Here's the drawing with two shaded views (mm, measured from the low corner). I have some questions. A direction names the side the tool comes from. Round coordinates to 2 decimals unless told otherwise and drop trailing zeros. Order: outer loops, then holes, each group sorted by start corner. A loop starts at its lowest first (then second) coordinate and runs counter-clockwise, first axis right, second up.
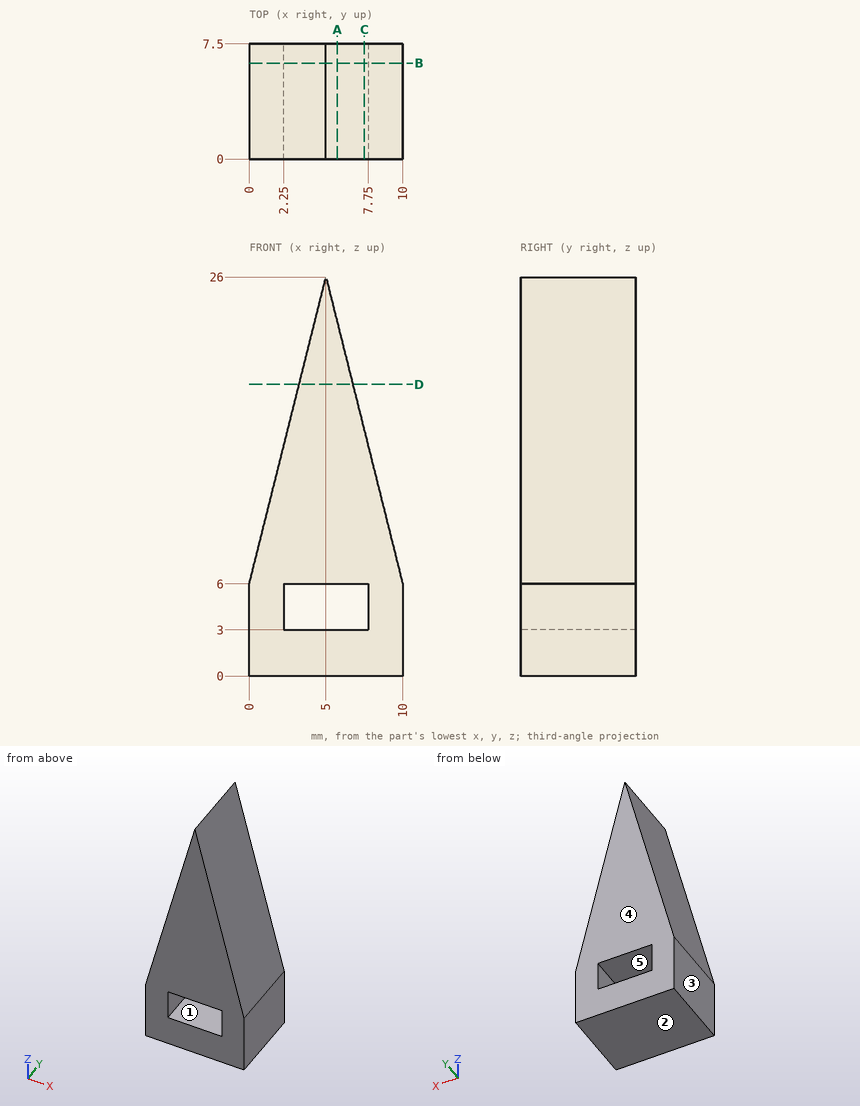
Q1. Imagine slicing it at A-A, the plane x = 5.75. Please give me the cut outline in (y, z), then the cut area to 3 significant figures.
Q2. I need wall thicknesses on L1, parallel to X at y = 5.75, z = 3.75; L2, parallel to X at y = 3.5, z = 15; L3, parallel to X at y = 1.25, z = 9.25. Which ranges of each line are inside material? Lowest first, please.
Q3. Imagine slicing it at D-D, the plane z = 19. Please give me the cut outline in (x, y).
Q4. We'd pull the mould along X, two halves only. Please class the marked faces 3, 4 and 5: released by +X, released by -X, zero draft, split by the parting line, or undercut.
Q5. For the marked faces 1 and 2, which set-ups out of +Z, -Z, +X, -X, +Y, -Y let a thin tool reach every point of the face, with its end or its side?
Q6. Imagine slicing it at B-B, the plane y = 6.25. Please give me the cut outline in (x, z).
Q7. Imagine slicing it at C-C, the plane x = 7.5. Please give me the cut outline in (y, z).
Q8. For P1, Ø1.5, axis at y = 4.5, z = 20, coming from the -X side, with a flat end and sliding along its axis, tell me the tip position at first contact or that it passes through.
Filled in:
1. outline: (0, 0) - (7.5, 0) - (7.5, 3) - (0, 3) - close; (0, 6) - (7.5, 6) - (7.5, 23) - (0, 23) - close
1. area: 150 mm2
2. L1: x = 0 to 2.25, 7.75 to 10
2. L2: x = 2.25 to 7.75
2. L3: x = 0.81 to 9.19
3. outline: (3.25, 0) - (6.75, 0) - (6.75, 7.5) - (3.25, 7.5) - close
4. face 3: released by -X
4. face 4: zero draft
4. face 5: undercut
5. face 1: +Y, -Y
5. face 2: -Z, +X, -X, +Y, -Y
6. outline: (0, 0) - (10, 0) - (10, 6) - (5, 26) - (0, 6) - close; hole (2.25, 3) - (7.75, 3) - (7.75, 6) - (2.25, 6) - close
7. outline: (0, 0) - (7.5, 0) - (7.5, 3) - (0, 3) - close; (0, 6) - (7.5, 6) - (7.5, 16) - (0, 16) - close
8. P1: stops at x = 3.31
